Verification items for the finished model (mm, model axes). A direction names the side the tool comes from. Give positions to 0.01 mm unless a question says otherwise; leave off trailing zeros. Write each loop counter-clockwise with the first axis right and the second up, starting at its lowest first coordinate (ties: lowest second). Pieces come first, ordered by that corner, then holes. Notation, with made-up numbers: (-31.75, -4) - (9.25, -4) arc R29 cw to (9.25, 35) - close; hole circle Ø1 at (-12.5, 30.25). An arc over 180 degrees is marked (long way). Answer as a JSON object with one key per item and string values. Group by question number.
Item 1: Sectioned sample at D-D, the plane x = -4. Record the boundary of the cut face in (y, z), and give its area (3 significant figures).
Item 2: Draft check along X on faces 5 (the face through (-7.171, -5.516, 44.671)), 6 (the face through (-6.157, -18, 25)), 7 (the face through (-42.84, 20.58, 46.9)). Enter one of: +X half, -X half, draft (parallel to the pull), parting line (faces both ways), or undercut.
Item 3: Tool access check on faces 1 (the face through (-29, 35.181, 25)), 2 (the face through (-64.843, 24.877, 47.993)), 3 (the face through (1.843, -11, 25)), 4 (the face through (-14.171, 20.544, 46.269)). Record the directions out of +Z, -Z, +X, -X, +Y, -Y that give a thin tool (end or side, any length) a straight path to the whole face; none if there is none.
Item 4: Sectioned sample at B-B, the plane y = 11.5. Record the boundary of the cut face in (x, z), and give its area (3 significant figures).
Item 5: Scan lines: line 1 along Y through (x, z) = (-53, 8); line 2 along Y through (x, z) = (-15, 29.5); line 3 along Y through (x, z) = (-11.5, 9.5). Record each from-to range of solid material in increasing order. Write a range as [from, to].
Item 6: Go/stop test with flat-tipped pins: pin 1 (20.5 mm diameter, centred on y = 25.5, z = 22, fed in from +X); pin 2 (3 mm diameter, centred on x = -6.5, z = 16.5, fed in from -Y); pin 3 (1.2 mm diameter, centred on x = -11.5, z = 34.5, fed in from -Y). Record where each tip stops, or that it passes through.
Item 7: Sectioned sample at C-C, the plane z = 23. Count the separate pieces of the cut face and the enclosed holes in it, and give its area (3 significant figures).
Item 8: Sectioned sample at A-A, the plane x = -59. Record the boundary of the cut face in (y, z), and give its area (3 significant figures).
```python
from build123d import *

# Parameters (mm, degrees)
CROQUIS3_W                  = 26.7
CROQUIS3_H                  = 26.7
CROQUIS3_W_2                = 4
CROQUIS3_H_2                = 25.7
CROQUIS3_W_3                = 13.5
CROQUIS3_H_3                = 3.969798642
SALIENTE_EXTRUIR1_DEPTH     = 50
SALIENTE_EXTRUIR2_DEPTH     = 50
CORTAR_EXTRUIR12_REACH      = 94.009
CORTAR_EXTRUIR13_REACH      = 79.272
CROQUIS13_W                 = 48
CROQUIS13_H                 = 15
REDONDEO1_R                 = 2.5
CORTAR_EXTRUIR14_REACH      = 88.292
REDONDEO2_R                 = 2.5
CORTAR_EXTRUIR15_REACH      = 92.548
REDONDEO3_R                 = 5
REDONDEO4_DEPTH             = 50
CORTAR_EXTRUIR17_REACH      = 81.89
CORTAR_EXTRUIR17_END_RADIUS = 16.15
REDONDEO5_R                 = 7
CORTAR_EXTRUIR18_REACH      = 92.661


with BuildPart() as part:
    # Croquis3 → Saliente-Extruir1 (new body)
    with BuildSketch(Plane.XY):
        with BuildLine():
            Line((-63.857247249, 32.580922569), (-63.857247249, 18.580922369))
            Line((-63.857247249, 18.580922369), (-43.857247249, 18.580922369))
            Line((-43.857247249, 18.580922369), (-43.857247249, 37.180922369))
            Line((-43.857247249, 37.180922369), (-27.007247249, 37.180922369))
            Line((-27.007247249, 37.180922369), (-6.157247249, 37.180922369))
            Line((-6.157247249, 37.180922369), (-6.157247249, -22.679560551))
            Line((-6.157247249, -22.679560551), (-26.590955846, -27.481197975))
            ThreePointArc((-26.590955846, -27.481197975), (-45.398833914, -17.697170572), (-42.099195701, 3.245032209))
            Line((-42.099195701, 3.245032209), (-42.099195701, 7.480922369))
            Line((-42.099195701, 7.480922369), (-43.857247249, 7.480922369))
            Line((-43.857247249, 7.480922369), (-43.857247249, 10.580922369))
            Line((-43.857247249, 10.580922369), (-65.856221771, 10.580922369))
            Line((-65.856221771, 10.580922369), (-65.856221771, 16.580922369))
            Line((-65.856221771, 16.580922369), (-65.856221771, 32.580922569))
            Line((-65.856221771, 32.580922569), (-63.857247249, 32.580922569))
        make_face()
        with Locations((-28.507247249, 21.830922369)):
            Rectangle(CROQUIS3_W, CROQUIS3_H, mode=Mode.SUBTRACT)
        with Locations((-11.157247249, 22.330922369)):
            Rectangle(CROQUIS3_W_2, CROQUIS3_H_2, mode=Mode.SUBTRACT)
        with Locations((-50.607247249, 14.56582169)):
            Rectangle(CROQUIS3_W_3, CROQUIS3_H_3, mode=Mode.SUBTRACT)
        with BuildLine():
            Line((-8.157247249, 2.82108494), (-26.731262437, 6.441781026))
            ThreePointArc((-26.731262437, 6.441781026), (-45.345288804, -9.402744466), (-26.961453667, -25.513783269))
            Line((-26.961453667, -25.513783269), (-8.157247249, -21.095056202))
            Line((-8.157247249, -21.095056202), (-8.157247249, 2.82108494))
        make_face(mode=Mode.SUBTRACT)
    extrude(amount=SALIENTE_EXTRUIR1_DEPTH)

    # Croquis11 → Saliente-Extruir2 (add)
    with BuildSketch(Plane(origin=(0, 0, 0), x_dir=(-1, 0, 0), z_dir=(0, 0, -1))):
        Polygon((-1.842752751, -14.302804028), (-1.842752751, -0.302804028), (6.157247249, -0.302804028), (6.157247249, -2.302804028), (2.157247249, -2.302804028), (2.157247249, -12.302804028), (6.157247249, -12.302804028), (6.157247249, -14.302804028), align=None)
    extrude(amount=-SALIENTE_EXTRUIR2_DEPTH)

    # Cortar-Extruir12: up to this face of the body (flat: up to its plane)
    cortar_extruir12_end = Plane(part.part.faces().sort_by_distance((-8.157247249, -9.136985631, 25))[0])
    # Croquis12 → Cortar-Extruir12 (cut, up to the picked face)
    with BuildSketch(Plane(origin=(1.842752751, 0, 0), x_dir=(0, 0, -1), z_dir=(1, 0, 0)), mode=Mode.PRIVATE) as cortar_extruir12_sk1:
        Polygon((-25, -9.802804028), (-4.8, -9.802804028), (-4.8, -4.802804028), (-45.42287301, -4.802804028), (-45.42287301, -9.802804028), align=None)
    cortar_extruir12_tool1 = split(extrude(cortar_extruir12_sk1.sketch, amount=-CORTAR_EXTRUIR12_REACH, mode=Mode.PRIVATE), bisect_by=cortar_extruir12_end, keep=Keep.BOTH, mode=Mode.PRIVATE)
    add(cortar_extruir12_tool1.solids().sort_by(Axis((1.842753, -7.302804, 25.111437), (-1, 0, 0)))[0], mode=Mode.SUBTRACT)

    # Croquis13 → Cortar-Extruir13 (cut, up to next)
    with BuildSketch(Plane.ZY.offset(43.857247249), mode=Mode.PRIVATE) as cortar_extruir13_sk1:
        with Locations((25, 26.080922369)):
            Rectangle(CROQUIS13_W, CROQUIS13_H)
    cortar_extruir13_tool1 = extrude(cortar_extruir13_sk1.sketch, amount=-CORTAR_EXTRUIR13_REACH, mode=Mode.PRIVATE) & part.part
    add(cortar_extruir13_tool1.solids().sort_by_distance((-43.857247, 26.080922, 25))[0], mode=Mode.SUBTRACT)

    # Redondeo1
    redondeo1_edges = [part.edges().sort_by_distance(p)[0] for p in [
        (-0.157247249, -4.802804028, 4.8),
        (-0.157247249, -9.802804028, 4.8),
        (-0.157247249, -9.802804028, 45.42287301),
        (-0.157247249, -4.802804028, 45.42287301),
        (-7.157247249, -9.802804028, 4.8),
        (-7.157247249, -4.802804028, 4.8),
        (-7.157247249, -9.802804028, 45.42287301),
        (-7.157247249, -4.802804028, 45.42287301),
    ]]
    fillet(redondeo1_edges, radius=REDONDEO1_R - 0.0001)  # a hair under: the kernel refuses the full size

    # Cortar-Extruir14: up to this face of the body (flat: up to its plane)
    cortar_extruir14_end = Plane(part.part.faces().sort_by_distance((-15.157247249, 21.830922369, 25))[0])
    # Croquis14 → Cortar-Extruir14 (cut, up to the picked face)
    with BuildSketch(Plane(origin=(-6.157247249, 0, 0), x_dir=(0, 0, -1), z_dir=(1, 0, 0)), mode=Mode.PRIVATE) as cortar_extruir14_sk1:
        Polygon((-2.979356026, 22.330922369), (-2.979356026, 19.830922369), (-47.020643974, 19.830922369), (-47.020643974, 22.330922369), (-47.020643974, 24.830922369), (-2.979356026, 24.830922369), align=None)
    cortar_extruir14_tool1 = split(extrude(cortar_extruir14_sk1.sketch, amount=-CORTAR_EXTRUIR14_REACH, mode=Mode.PRIVATE), bisect_by=cortar_extruir14_end, keep=Keep.BOTH, mode=Mode.PRIVATE)
    add(cortar_extruir14_tool1.solids().sort_by(Axis((-6.157247, 22.330922, 25), (-1, 0, 0)))[0], mode=Mode.SUBTRACT)

    # Redondeo2
    redondeo2_edges = [part.edges().sort_by_distance(p)[0] for p in [
        (-14.157247249, 24.830922369, 2.979356026),
        (-7.657247249, 24.830922369, 2.979356026),
        (-7.657247249, 19.830922369, 2.979356026),
        (-14.157247249, 19.830922369, 2.979356026),
        (-14.157247249, 24.830922369, 47.020643974),
        (-7.657247249, 24.830922369, 47.020643974),
        (-7.657247249, 19.830922369, 47.020643974),
        (-14.157247249, 19.830922369, 47.020643974),
    ]]
    fillet(redondeo2_edges, radius=REDONDEO2_R - 0.0001)  # a hair under: the kernel refuses the full size

    # Croquis15 → Cortar-Extruir15 (cut, up to next)
    with BuildSketch(Plane(origin=(-63.857247249, 0, 0), x_dir=(0, 0, -1), z_dir=(1, 0, 0)), mode=Mode.PRIVATE) as cortar_extruir15_sk1:
        with BuildLine():
            Line((-31, 26.080922569), (-19, 26.080922569))
            Line((-19, 26.080922569), (-13.809474968, 26.080922569))
            ThreePointArc((-13.809474968, 26.080922569), (-2.023506642, 25.111513684), (-13.454356149, 22.080922569))
            Line((-13.454356149, 22.080922569), (-19, 22.080922569))
            Line((-19, 22.080922569), (-31, 22.080922569))
            Line((-31, 22.080922569), (-36.545643851, 22.080922569))
            ThreePointArc((-36.545643851, 22.080922569), (-47.976493358, 25.111513684), (-36.190525032, 26.080922569))
            Line((-36.190525032, 26.080922569), (-31, 26.080922569))
        make_face()
    cortar_extruir15_tool1 = extrude(cortar_extruir15_sk1.sketch, amount=-CORTAR_EXTRUIR15_REACH, mode=Mode.PRIVATE) & part.part
    add(cortar_extruir15_tool1.solids().sort_by_distance((-63.857247, 24.436716, 25))[0], mode=Mode.SUBTRACT)

    # Redondeo3
    redondeo3_edges = [part.edges().sort_by_distance(p)[0] for p in [
        (-65.856221771, 10.580922369, 25),
    ]]
    fillet(redondeo3_edges, radius=REDONDEO3_R)

    # Redondeo4: read off the stored shape, not the designer's step
    # Redondeo4 outline → Redondeo4 (add)
    with BuildSketch(Plane.XY):
        with BuildLine():
            Line((-42.099195701, 7.480922369), (-43.857247249, 7.480922369))
            add(Edge.make_bspline(
                [(-43.857247249, 7.480922369), (-42.099195701, 6.934552825), (-42.099195701, 5.093557191)],
                knots=[0, 0, 0, 1, 1, 1], degree=2, weights=[1, 0.402613242, 1]))
            Line((-42.099195701, 5.093557191), (-42.099195701, 7.480922369))
        make_face()
    extrude(amount=REDONDEO4_DEPTH)

    # Cortar-Extruir17: up to this cylinder (the profile starts outside it)
    cortar_extruir17_end = Plane(origin=(-29.1957078, -9.519077631, 25), z_dir=(0, 0, -1)) * Cylinder(CORTAR_EXTRUIR17_END_RADIUS, 197.08, mode=Mode.PRIVATE)
    # Croquis16 → Cortar-Extruir17 (cut, up to the surface)
    with BuildSketch(Plane.ZY.offset(48.157247249), mode=Mode.PRIVATE) as cortar_extruir17_sk1:
        with BuildLine():
            Line((32, -25.481197975), (18, -25.481197975))
            ThreePointArc((18, -25.481197975), (8.807611845, -21.67358613), (5, -12.481197975))
            Line((5, -12.481197975), (5, -11.754967791))
            ThreePointArc((5, -11.754967791), (8.807611845, -2.562579636), (18, 1.245032209))
            Line((18, 1.245032209), (32, 1.245032209))
            ThreePointArc((32, 1.245032209), (41.192388155, -2.562579636), (45, -11.754967791))
            Line((45, -11.754967791), (45, -12.481197975))
            ThreePointArc((45, -12.481197975), (41.192388155, -21.67358613), (32, -25.481197975))
        make_face()
    cortar_extruir17_tool1 = extrude(cortar_extruir17_sk1.sketch, amount=-CORTAR_EXTRUIR17_REACH, mode=Mode.PRIVATE) - cortar_extruir17_end
    add(cortar_extruir17_tool1.solids().sort_by_distance((-48.157247, -12.118083, 25))[0], mode=Mode.SUBTRACT)

    # Redondeo5
    redondeo5_edges = [part.edges().sort_by_distance(p)[0] for p in [
        (-42.857247249, 18.580922369, 1),
        (-42.857247249, 33.580922369, 1),
        (-42.857247249, 33.580922369, 49),
        (-42.857247249, 18.580922369, 49),
    ]]
    fillet(redondeo5_edges, radius=REDONDEO5_R)

    # Croquis17 → Cortar-Extruir18 (cut, up to next)
    with BuildSketch(Plane(origin=(0, 0, 0), x_dir=(-1, 0, 0), z_dir=(0, 0, -1)), mode=Mode.PRIVATE) as cortar_extruir18_sk1:
        with BuildLine():
            Line((60.856221771, 12.580922369), (57.357247249, 12.580922369))
            Line((57.357247249, 12.580922369), (57.357247249, 16.550721011))
            Line((57.357247249, 16.550721011), (63.856221771, 16.550721011))
            Line((63.856221771, 16.550721011), (63.856221771, 15.580922369))
            ThreePointArc((63.856221771, 15.580922369), (62.977542115, 13.459602026), (60.856221771, 12.580922369))
        make_face()
    cortar_extruir18_tool1 = extrude(cortar_extruir18_sk1.sketch, amount=-CORTAR_EXTRUIR18_REACH, mode=Mode.PRIVATE) & part.part
    add(cortar_extruir18_tool1.solids().sort_by_distance((-60.398011, 14.672215, 0))[0], mode=Mode.SUBTRACT)


solid = part.part
```
Geometry check:
{
 "1": {"outline": "(-14.3, 0) - (-12.3, 0) - (-12.3, 50) - (-14.3, 50) - close; (-2.3, 0) - (-0.3, 0) - (-0.3, 50) - (-2.3, 50) - close", "area": "200 mm^2"},
 "2": {"face 5": "draft", "face 6": "+X half", "face 7": "undercut"},
 "3": {"face 1": "+Z, -Z", "face 2": "-X", "face 3": "+Z, -Z, +X, +Y, -Y", "face 4": "+X, -X"},
 "4": {"outline": "(-63.75, 0) - (-41.86, 0) - (-41.86, 50) - (-63.75, 50) - close; (-15.16, 0) - (-13.16, 0) - (-13.16, 50) - (-15.16, 50) - close; (-9.16, 0) - (-6.16, 0) - (-6.16, 50) - (-9.16, 50) - close", "area": "1,340 mm^2"},
 "5": {"line 1": "[10.58, 12.58], [16.55, 18.58]", "line 2": "[-24.76, -22.7], [4.15, 19.83], [24.83, 37.18]", "line 3": "[-23.94, -21.88], [3.47, 9.48], [35.18, 37.18]"},
 "6": {"pin 1": "x = -6.16", "pin 2": "y = -23.11", "pin 3": "y = -24.08"},
 "7": {"separate pieces": "4", "enclosed holes": "1", "area": "614 mm^2"},
 "8": {"outline": "(10.58, 0) - (12.58, 0) - (12.58, 50) - (10.58, 50) - close; (16.55, 0) - (18.58, 0) - (18.58, 50) - (16.55, 50) - close", "area": "202 mm^2"}
}
